Geometry: final body of the model. Coordinates: model frame, mm. Face numbers are marked on the shaded views. A direction names the side the tool comes from. Coordinates: 2 decimals unless noted, no trailing zeros. Loops run counter-clockwise (first coordinate to the right, second up) from the corner with the lowest first, then second, coordinate; pieces in that order, holes last. Notation, with made-up numbers: (0, 83.25) - (7, 83.25) arc R11 ccw to (7, 95.25) - close; hole circle Ø6 at (41, 74). An arc over 180 degrees is marked (long way). Put each result on its own line as item: value. Start each with the question number.
1) Section A-A on x = 0. Output: boundary loops of the cut face in (y, z).
2) Section B-B on y = 7. Output: boundary loops of the cut face in (x, z), and give its area (3 significant figures).
3) Section C-C on x = 15. Count the separate pieces of the cut face and the enclosed holes in it, and give its area (3 significant figures).
4) Reachability of the marked faces 5, 6 and 7 from +Z, -Z, +X, -X, +Y, -Y: full face, straight path, thin tool, end or side. Return the list, or none.
5) Material intervals for line 1 along X through (y, z) = (3.7, 0); line 2 along X through (y, z) = (26.5, 12), sorted ascending. Write a range as from..to.
6) Section D-D on z = 0. Output: boundary loops of the cut face in (x, y).
7) Draft query along Z for the marked faces 1, 2, 3 and 4. Return one class per face: +Z half, -Z half, draft (parallel to the pull), parting line (faces both ways), or undercut.
8) Contact query for flat-ended pins moving along their axis: pin 1 Ø3 at (x, z) = (9.525, 0) entering from +Y; pin 2 Ø8 at (x, z) = (-4.5, 3) entering from +Y; pin 3 Ø6 at (x, z) = (2, 15.5) entering from +Y. Output: stop coordinate, or through.
```python
from build123d import *

# Parameters (mm, degrees)
SKETCH1_W           = 26.035
SKETCH1_H           = 26.035
SKETCH1_R           = 1.778
BOSS_EXTRUDE1_DEPTH = 5.08
SKETCH9_W           = 41.275
SKETCH9_H           = 41.275
SKETCH9_W_2         = 26.035
SKETCH9_H_2         = 26.035
BOSS_EXTRUDE7_DEPTH = 38.1
CUT_EXTRUDE4_DEPTH  = 42.275
SKETCH11_R          = 3.175
CUT_EXTRUDE5_DEPTH  = 42.275
FILLET1_R           = 3.81
FILLET2_R           = 3.81


with BuildPart() as part:
    # Sketch1 → Boss-Extrude1 (new body)
    with BuildSketch(Plane(origin=(0, 0, 0), x_dir=(1, 0, 0), z_dir=(0, 1, 0))):
        Rectangle(SKETCH1_W, SKETCH1_H)
        with Locations((0, 9.525)):
            Circle(SKETCH1_R, mode=Mode.SUBTRACT)
        with Locations((-9.525, 0)):
            Circle(SKETCH1_R, mode=Mode.SUBTRACT)
        with Locations((9.525, 0)):
            Circle(SKETCH1_R, mode=Mode.SUBTRACT)
        with Locations((0, -9.525)):
            Circle(SKETCH1_R, mode=Mode.SUBTRACT)
    extrude(amount=BOSS_EXTRUDE1_DEPTH)

    # Sketch9 → Boss-Extrude7 (add)
    with BuildSketch(Plane.XZ):
        Rectangle(SKETCH9_W, SKETCH9_H)
        Rectangle(SKETCH9_W_2, SKETCH9_H_2, mode=Mode.SUBTRACT)
    extrude(amount=-BOSS_EXTRUDE7_DEPTH)

    # Sketch10 → Cut-Extrude4 (cut, through all)
    with BuildSketch(Plane.XY.offset(20.6375)):
        with BuildLine():
            Line((-13.0175, 20.32), (-13.0175, 38.1))
            Line((-13.0175, 38.1), (13.0175, 38.1))
            Line((13.0175, 38.1), (13.0175, 20.32))
            ThreePointArc((13.0175, 20.32), (10.785653673, 14.931846327), (5.3975, 12.7))
            Line((5.3975, 12.7), (-5.3975, 12.7))
            ThreePointArc((-5.3975, 12.7), (-10.785653673, 14.931846327), (-13.0175, 20.32))
        make_face()
    extrude(amount=-CUT_EXTRUDE4_DEPTH, mode=Mode.SUBTRACT)

    # Sketch11 → Cut-Extrude5 (cut, through all)
    with BuildSketch(Plane.ZY.offset(20.6375)):
        with Locations((-9.525, 30.48)):
            Circle(SKETCH11_R)
        with Locations((9.525, 30.48)):
            Circle(SKETCH11_R)
    extrude(amount=-CUT_EXTRUDE5_DEPTH, mode=Mode.SUBTRACT)

    # Fillet1
    fillet1_edges = [part.edges().sort_by_distance(p)[0] for p in [
        (20.6375, 19.05, -20.6375),
        (-20.6375, 19.05, -20.6375),
        (-20.6375, 19.05, 20.6375),
        (20.6375, 19.05, 20.6375),
    ]]
    fillet(fillet1_edges, radius=FILLET1_R)

    # Fillet2
    fillet2_edges = [part.edges().sort_by_distance(p)[0] for p in [
        (0, 0, -20.6375),
        (20.6375, 0, 0),
        (0, 0, 20.6375),
        (-20.6375, 0, 0),
        (-19.521576836, 0, 19.521576836),
        (-19.521576836, 0, -19.521576836),
        (19.521576836, 0, 19.521576836),
        (19.521576836, 0, -19.521576836),
    ]]
    fillet(fillet2_edges, radius=FILLET2_R)


solid = part.part
```
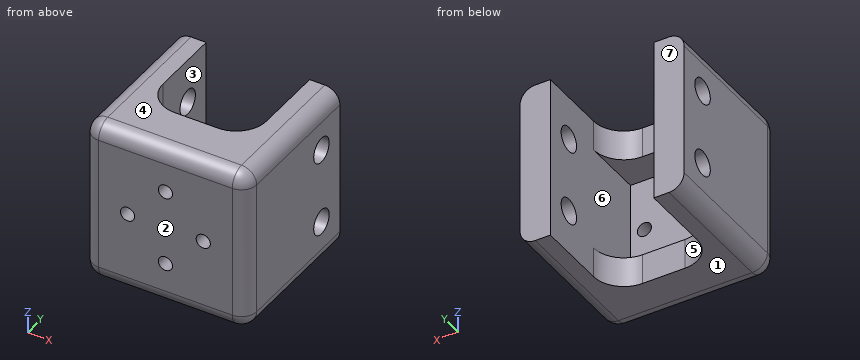
Answer block:
1. outline: (0, -16.83) arc R3.81 ccw to (3.81, -20.64) - (12.7, -20.64) - (12.7, -13.02) - (5.08, -13.02) - (5.08, -11.3) - (0, -11.3) - close; (0, -7.75) - (5.08, -7.75) - (5.08, 7.75) - (0, 7.75) - close; (0, 11.3) - (5.08, 11.3) - (5.08, 13.02) - (12.7, 13.02) - (12.7, 20.64) - (3.81, 20.64) arc R3.81 ccw to (0, 16.83) - close
2. outline: (-20.64, -16.83) arc R3.81 ccw to (-16.83, -20.64) - (16.83, -20.64) arc R3.81 ccw to (20.64, -16.83) - (20.64, 16.83) arc R3.81 ccw to (16.83, 20.64) - (-16.83, 20.64) arc R3.81 ccw to (-20.64, 16.83) - close; hole (-13.02, -13.02) - (13.02, -13.02) - (13.02, 13.02) - (-13.02, 13.02) - close
2. area: 1,010 mm²
3. separate pieces: 1
3. enclosed holes: 2
3. area: 1,500 mm²
4. face 5: +Z, -Z, +Y
4. face 6: +Y
4. face 7: +Z, -Z, +X, -X, +Y
5. line 1: x = -20.64..-11.3, -7.75..7.75, 11.3..20.64
5. line 2: x = -20.64..-13.02, 13.02..20.64
6. outline: (-20.64, 3.81) arc R3.81 ccw to (-16.83, 0) - (-11.3, 0) - (-11.3, 5.08) - (-13.02, 5.08) - (-13.02, 38.1) - (-20.64, 38.1) - close; (-7.75, 0) - (7.75, 0) - (7.75, 5.08) - (-7.75, 5.08) - close; (11.3, 0) - (16.83, 0) arc R3.81 ccw to (20.64, 3.81) - (20.64, 38.1) - (13.02, 38.1) - (13.02, 5.08) - (11.3, 5.08) - close
7. face 1: -Z half
7. face 2: draft
7. face 3: undercut
7. face 4: +Z half
8. pin 1: passes through
8. pin 2: stops at y = 5.08
8. pin 3: stops at y = 12.7
